The figure shows three views and two pictorial views of one solid part (mm, origin at its lowest corner). Answer the questions. Round coordinates to 2 decimals unless told otherwise and drop trailing zeros. Order: outer loops, then holes, each group sorted by start corner. A loop starts at its lowest first (then second) coordinate and runs counter-clockwise, first axis right, second up. Notation, with made-up numbers: (31, 5.5) - (48, 5.5) arc R17 ccw to (48, 21.5) - close; hole circle Ø9 at (67.25, 10.5). An arc over 180 degrees is marked (long way). Answer as a JSON object with one key per item and string values. Group by question number.
Q1. Given pin 1 Ø2.5 at (x, z) = (5.55, 36.65) entering from -Y, flat-ended and moving along its own axis, determine where the tip first touches the part or whether it passes through.
Q2. A cutting plane is placed at C-C on y = 18. Determine the outline of the cut face in (x, z).
Q3. A cutting plane is placed at B-B on z = 36.65. Determine the outline of the cut face in (x, y).
Q4. Consider line 1 (Z direction, x = 36.65, y = 10); line 2 (X direction, y = 25, z = 36.5); line 3 (X direction, y = 22.5, z = 36). Determine where each line is inside the solid, lowest interval first.
Q5. A cutting plane is placed at A-A on x = 5.55. Determine the outline of the cut face in (y, z), and give its area (3 significant figures).
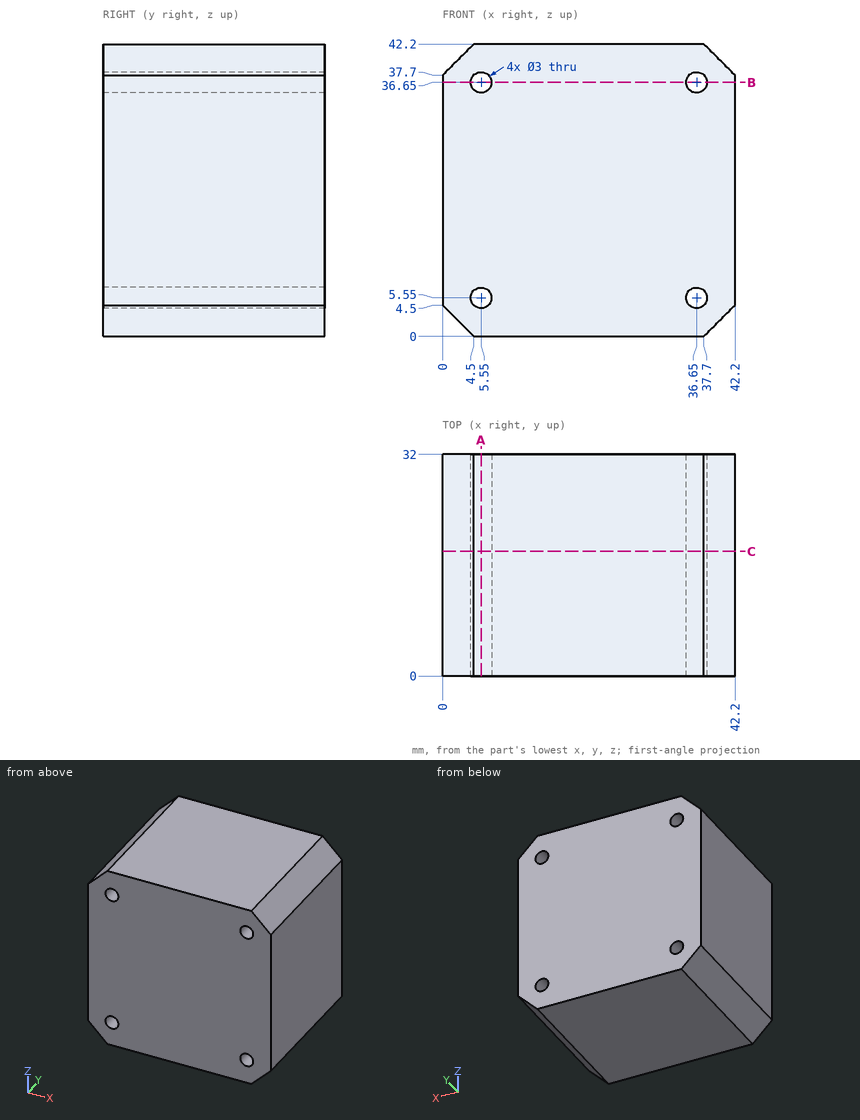
Result set:
{
 "1": {"pin 1": "passes through"},
 "2": {"outline": "(0, 4.5) - (4.5, 0) - (37.7, 0) - (42.2, 4.5) - (42.2, 37.7) - (37.7, 42.2) - (4.5, 42.2) - (0, 37.7) - close; hole circle Ø3 at (5.55, 5.55); hole circle Ø3 at (5.55, 36.65); hole circle Ø3 at (36.65, 5.55); hole circle Ø3 at (36.65, 36.65)"},
 "3": {"outline": "(0, 0) - (4.05, 0) - (4.05, 32) - (0, 32) - close; (7.05, 0) - (35.15, 0) - (35.15, 32) - (7.05, 32) - close; (38.15, 0) - (42.2, 0) - (42.2, 32) - (38.15, 32) - close"},
 "4": {"line 1": "z = 0 to 4.05, 7.05 to 35.15, 38.15 to 42.2", "line 2": "x = 0 to 4.06, 7.04 to 35.16, 38.14 to 42.2", "line 3": "x = 0 to 4.2, 6.9 to 35.3, 38 to 42.2"},
 "5": {"outline": "(0, 0) - (32, 0) - (32, 4.05) - (0, 4.05) - close; (0, 7.05) - (32, 7.05) - (32, 35.15) - (0, 35.15) - close; (0, 38.15) - (32, 38.15) - (32, 42.2) - (0, 42.2) - close", "area": "1,160 mm²"}
}
